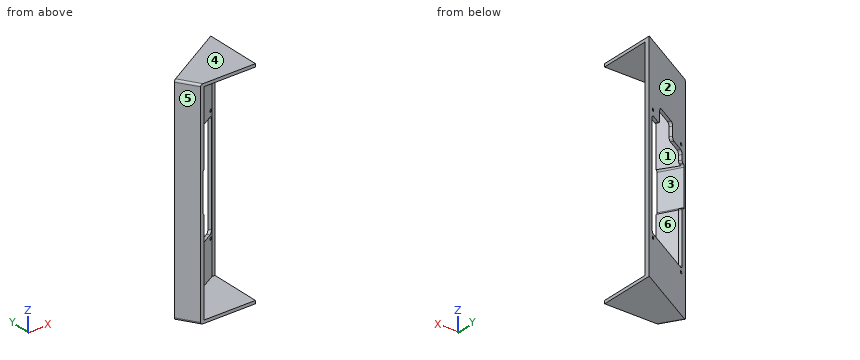
from build123d import *

# Parameters (mm, degrees)
BOSS_EXTRUDE1_DEPTH = 3
BOSS_EXTRUDE2_DEPTH = 208
BOSS_EXTRUDE4_DEPTH = 3
SKETCH3_R           = 1.375
PIHOLE_DEPTH        = 33.822362803
PIHOLE_DEPTH_BACK   = 49.737803669
CUT_EXTRUDE7_START  = -3
SKETCH11_W          = 3
SKETCH11_H          = 51.081415713
CUT_EXTRUDE7_DEPTH  = 208
FILLET1_R           = 2


with BuildPart() as part:
    # Sketch1 → Boss-Extrude1 (new body)
    with BuildSketch(Plane.XY):
        Polygon((131.589833852, 656.464158154), (185.834178461, 656.464158154), (185.834178461, 712.741726289), (120.189452854, 674.841726289), align=None)
    extrude(amount=BOSS_EXTRUDE1_DEPTH)

    # Sketch2 → Boss-Extrude2 (add)
    with BuildSketch(Plane.XY):
        Polygon((185.834178461, 712.741726289), (120.189452854, 674.841726289), (131.589833852, 656.464158154), (135.120190771, 656.464158154), (124.371071621, 673.791883395), (182.834178461, 707.545573867), (182.834178461, 656.464158154), (185.834178461, 656.464158154), align=None)
    extrude(amount=-BOSS_EXTRUDE2_DEPTH)

    # Sketch10 → Boss-Extrude4 (add)
    with BuildSketch(Plane(origin=(0, 0, -208), x_dir=(-1, 0, 0), z_dir=(0, 0, -1))):
        Polygon((-185.834178461, 712.741726289), (-120.189452854, 674.841726289), (-131.589833852, 656.464158154), (-185.834178461, 656.464158154), align=None)
    extrude(amount=BOSS_EXTRUDE4_DEPTH)

    # Sketch3 → PiHole (cut, two sides)
    with BuildSketch(Plane(origin=(-262.167676037, 454.087734998, 0), x_dir=(0.866025404, 0.5, 0), z_dir=(-0.5, 0.866025404, 0))) as pihole_sk:
        with Locations((450.507982584, 172.9)):
            Circle(SKETCH3_R)
        with Locations((509.607982584, 172.9)):
            Circle(SKETCH3_R)
        with Locations((509.607982584, 58.9)):
            Circle(SKETCH3_R)
        with Locations((450.507982584, 58.9)):
            Circle(SKETCH3_R)
        with BuildLine():
            Line((451.507982584, 169), (508.307982584, 169))
            ThreePointArc((508.307982584, 169), (510.429302927, 168.121320344), (511.307982584, 166))
            Line((511.307982584, 166), (511.307982584, 67))
            ThreePointArc((511.307982584, 67), (510.429302927, 64.878679656), (508.307982584, 64))
            Line((508.307982584, 64), (498.307982584, 64))
            ThreePointArc((498.307982584, 64), (496.18666224, 63.121320344), (495.307982584, 61))
            Line((495.307982584, 61), (495.307982584, 52))
            ThreePointArc((495.307982584, 52), (494.429302927, 49.878679656), (492.307982584, 49))
            Line((492.307982584, 49), (471.507982584, 49))
            ThreePointArc((471.507982584, 49), (469.38666224, 49.878679656), (468.507982584, 52))
            Line((468.507982584, 52), (468.507982584, 61))
            ThreePointArc((468.507982584, 61), (467.629302927, 63.121320344), (465.507982584, 64))
            Line((465.507982584, 64), (451.507982584, 64))
            ThreePointArc((451.507982584, 64), (449.38666224, 64.878679656), (448.507982584, 67))
            Line((448.507982584, 67), (448.507982584, 72))
            ThreePointArc((448.507982584, 72), (447.922196146, 73.414213562), (446.507982584, 74))
            Line((446.507982584, 74), (446.007982584, 74))
            ThreePointArc((446.007982584, 74), (444.593769021, 74.585786438), (444.007982584, 76))
            Line((444.007982584, 76), (444.007982584, 112))
            ThreePointArc((444.007982584, 112), (444.593769021, 113.414213562), (446.007982584, 114))
            Line((446.007982584, 114), (446.507982584, 114))
            ThreePointArc((446.507982584, 114), (447.922196146, 114.585786438), (448.507982584, 116))
            Line((448.507982584, 116), (448.507982584, 166))
            ThreePointArc((448.507982584, 166), (449.38666224, 168.121320344), (451.507982584, 169))
        make_face()
    extrude(amount=PIHOLE_DEPTH, mode=Mode.SUBTRACT)
    extrude(pihole_sk.sketch, amount=-PIHOLE_DEPTH_BACK, mode=Mode.SUBTRACT)

    # Sketch11 → Cut-Extrude7 (cut)
    with BuildSketch(Plane.XY.offset(3).offset(CUT_EXTRUDE7_START)):
        with Locations((184.334178461, 682.004866011)):
            Rectangle(SKETCH11_W, SKETCH11_H)
    extrude(amount=-CUT_EXTRUDE7_DEPTH, mode=Mode.SUBTRACT)

    # Fillet1
    fillet1_edges = [part.edges().sort_by_distance(p)[0] for p in [
        (125.889643353, 665.652942222, 3),
        (125.889643353, 665.652942222, -211),
    ]]
    fillet(fillet1_edges, radius=FILLET1_R)


solid = part.part
Could you check a few things on this model? Use its own coordinates, in mm. Face numbers are marked on the shaded views. A direction names the side the tool comes from. Round coordinates to 2 decimals unless told otherwise and drop trailing zeros. Write each loop counter-clockwise with the first axis right and the second up, starting at its lowest first coordinate (ties: lowest second). Pieces come first, ordered by that corner, then holes. Notation, with made-up numbers: (-7.5, 38) - (-0.5, 38) arc R16 cw to (-0.5, 63) - close; hole circle Ø8 at (25, 76.25). An arc over 180 degrees is marked (long way). Put each result on its own line as item: value. Start each with the question number.
(1) Thinking about a two-plate mould opening in Y: for the marked faces 4, 5 and 6, which applies, released by +Y, released by -Y, zero draft, split by the parting line, or undercut?
(2) I need wall thicknesses on probe 1 along Z at (x, y) = (183.5, 673.5); probe 2 along Y at (x, z) = (129.5, -21); probe 3 along Y at (x, z) = (128, -51.5). Which ranges of each line are inside material? Lowest first, please.
(3) For the marked faces 1, 2 and 3, which set-ups out of +Z, -Z, +X, -X, +Y, -Y let a thin tool reach every point of the face, with its end or its side?
(4) Will these pins go through, and if not, where does the flat tip stop? pin 1 (3 mm diameter, centred on y = 675, z = -138, fed in from -X); pin 2 (0.9 mm diameter, centred on x = 184, z = -69, fed in from -Y); pin 3 (8 mm diameter, centred on x = 150, z = -186, fed in from -Y).
(5) I want a section at B-B, the plane z = -47. Please give me the cut outline in (x, y), plus the area to 3 significant figures.
(6) I want a section at C-C, the plane z = -96. Please give me the cut outline in (x, y), plus the area to 3 significant figures.
(7) I want a section at A-A, the plane z = -151.5. Please give me the cut outline in (x, y).
Here are the results:
1. face 4: zero draft
1. face 5: released by -Y
1. face 6: undercut
2. probe 1: z = -211 to -208, 0 to 3
2. probe 2: y = 659.83 to 665.52, 676.75 to 680.22
2. probe 3: y = 662.25 to 667.94, 675.89 to 679.35
3. face 1: +X
3. face 2: +Z, -Z, -X, +Y
3. face 3: +X, +Y
4. pin 1: stops at x = 120.19
4. pin 2: stops at y = 707.55
4. pin 3: stops at y = 686.28
5. outline: (120.19, 674.84) - (131.59, 656.46) - (135.12, 656.46) - (124.37, 673.79) - (182.83, 707.55) - (185.83, 707.55) - (185.83, 712.74) - close
5. area: 286 mm^2
6. outline: (120.19, 674.84) - (131.59, 656.46) - (133.69, 656.46) - (122.35, 676.09) - close; (180.64, 709.74) - (182.14, 707.14) - (182.83, 707.55) - (185.83, 707.55) - (185.83, 712.74) - close
6. area: 65.6 mm^2
7. outline: (120.19, 674.84) - (131.59, 656.46) - (135.12, 656.46) - (124.37, 673.79) - (127.75, 675.74) - (126.25, 678.34) - close; (180.64, 709.74) - (182.14, 707.14) - (182.83, 707.55) - (185.83, 707.55) - (185.83, 712.74) - close
